```python
from build123d import *

# Parameters (mm, degrees)
F0_R     = 31.75
F1_DEPTH = 12.7
F2_R     = 3
F3_DEPTH = 12.701
F4_R     = 9.95
F5_DEPTH = 12.7
F7_DEPTH = 25.4
F8_R     = 9.525
F9_DEPTH = 19.05


with BuildPart() as f1:
    # F0 (on Top) → F1 (new body)
    with BuildSketch(Plane.XY):
        Circle(F0_R)
    extrude(amount=F1_DEPTH)

    # F2 (on face) → F3 (cut, through all)
    with BuildSketch(Plane.XY.offset(12.7)):
        with Locations((0, 22.5)):
            Circle(F2_R)
        with Locations((-19.485572, 11.25)):
            Circle(F2_R)
        with Locations((-19.485572, -11.25)):
            Circle(F2_R)
        with Locations((0, -22.5)):
            Circle(F2_R)
        with Locations((19.485572, -11.25)):
            Circle(F2_R)
        with Locations((19.485572, 11.25)):
            Circle(F2_R)
    extrude(amount=-F3_DEPTH, mode=Mode.SUBTRACT)

    # F4 (on face) → F5 (cut)
    with BuildSketch(Plane(origin=(0, 0, 0), x_dir=(1, 0, 0), z_dir=(0, 0, -1))):
        Circle(F4_R)
    extrude(amount=-F5_DEPTH, mode=Mode.SUBTRACT)

    # F6 (on face) → F7 (join)
    with BuildSketch(Plane.XY.offset(12.7)):
        with BuildLine():
            ThreePointArc((-4.030746, -18.055556), (0, -16.5), (4.030746, -18.055556))
            ThreePointArc((4.030746, -18.055556), (9.25, -16.02147), (13.621197, -12.518506))
            ThreePointArc((13.621197, -12.518506), (14.289419, -8.25), (17.651943, -5.537049))
            ThreePointArc((17.651943, -5.537049), (18.5, 0), (17.651943, 5.537049))
            ThreePointArc((17.651943, 5.537049), (14.289419, 8.25), (13.621197, 12.518506))
            ThreePointArc((13.621197, 12.518506), (9.25, 16.02147), (4.030746, 18.055556))
            ThreePointArc((4.030746, 18.055556), (0, 16.5), (-4.030746, 18.055556))
            ThreePointArc((-4.030746, 18.055556), (-9.25, 16.02147), (-13.621197, 12.518506))
            ThreePointArc((-13.621197, 12.518506), (-14.289419, 8.25), (-17.651943, 5.537049))
            ThreePointArc((-17.651943, 5.537049), (-18.5, 0), (-17.651943, -5.537049))
            ThreePointArc((-17.651943, -5.537049), (-14.289419, -8.25), (-13.621197, -12.518506))
            ThreePointArc((-13.621197, -12.518506), (-9.25, -16.02147), (-4.030746, -18.055556))
        make_face()
    extrude(amount=F7_DEPTH)

    # F8 (on face) → F9 (cut)
    with BuildSketch(Plane.XY.offset(38.1)):
        Circle(F8_R)
    extrude(amount=-F9_DEPTH, mode=Mode.SUBTRACT)


solid = f1.part
```
Geometry check sheet. Reference: the model listing, model coordinates, mm. A direction names the side the tool comes from. Give positions to 0.01 mm unless a question says otherwise; leave off trailing zeros. Order: outer loops, then holes, each group sorted by start corner. A loop starts at its lowest first (then second) coordinate and runs counter-clockwise, first axis right, second up. Notation, with made-up numbers: (-31.5, 16.5) - (24.5, 16.5) arc R17 cw to (24.5, 21.5) - close; hole circle Ø7 at (13, 28). An arc over 180 degrees is marked (long way). Answer in a Markdown table with one row per item. Add a question column.
Q1. Mould release check, pull along X, two halves, no side actions. Record for faces 4 (the cylindrical face through (14.26, -8.3, 25.22)), 5 (the cylindrical face through (-0.1, -16.5, 25.2)), 6 (the flat face through (-8, -7, 0)), 7 (the cylindrical face through (-22.483, 11.382, 6.439)): pulls with the +X half, pulls with the -X half, needs draft (parallel to the pull), parting line crosses it, or undercut.
Q2. Material ranges on probe 1 along Y at (x, z) = (0, 8.25); probe 2 along Y at (x, z) = (22, 9.5); probe 3 along Z at (x, y) = (13, 23.5), recorded low to high. Write a range as from..to.
Q3. Cross-section at C-C, the plane y = 22.5. Enter the section's corners in (x, z).
Q4. Cross-section at D-D, the plane y = 11.25. Enter the section's corners in (x, z), then the cut area to 3 significant figures.
Q5. Gauge pin test, flat ends, axial feed: pin 1 (6 mm diameter, centred on x = 1, y = -1, fed in from -Z); pin 2 (5 mm diameter, centred on x = -0.5, z = 24, fed in from -Y); pin 3 (7 mm diameter, centred on x = 19.49, y = 11.25, fed in from +Z). Record the tip position at first contact, or that the pin passes through.
Q6. Tool access check on faces 1 (the cylindrical face through (9.18, -16.06, 25.22)), 2 (the cylindrical face through (-7.9, 6.05, 6.26)), 3 (the cylindrical face through (-7.559, -5.796, 28.708)). Record the directions out of +Z, -Z, +X, -X, +Y, -Y that give a thin tool (end or side, any length) a straight path to the whole face; none if there is none.
Q7. Cross-section at B-B, the plane x = 0. Enter the section's corners in (y, z) (3 decimals), then the cut area to 3 significant figures.
Check values:
| question | item | result |
|---|---|---|
| 1 | face 4 | pulls with the +X half |
| 1 | face 5 | undercut |
| 1 | face 6 | needs draft |
| 1 | face 7 | undercut |
| 2 | probe 1 | y = -31.75..-25.5, -19.5..-9.95, 9.95..19.5, 25.5..31.75 |
| 2 | probe 2 | y = -22.89..-12.89, -9.61..9.61, 12.89..22.89 |
| 2 | probe 3 | z = 0..12.7 |
| 3 | outline | (-22.4, 0) - (-3, 0) - (-3, 12.7) - (-22.4, 12.7) - close; (3, 0) - (22.4, 0) - (22.4, 12.7) - (3, 12.7) - close |
| 4 | outline | (-29.69, 0) - (-22.49, 0) - (-22.49, 12.7) - (-29.69, 12.7) - close; (-16.49, 0) - (16.49, 0) - (16.49, 12.7) - (13.49, 12.7) - (13.49, 38.1) - (-13.49, 38.1) - (-13.49, 12.7) - (-16.49, 12.7) - close; (22.49, 0) - (29.69, 0) - (29.69, 12.7) - (22.49, 12.7) - close |
| 4 | area | 1,290 mm^2 |
| 5 | pin 1 | stops at z = 12.7 |
| 5 | pin 2 | stops at y = -17.3 |
| 5 | pin 3 | stops at z = 12.7 |
| 6 | face 1 | +Z, +X, -Y |
| 6 | face 2 | -Z |
| 6 | face 3 | +Z |
| 7 | outline | (-31.75, 0) - (-25.5, 0) - (-25.5, 12.7) - (-31.75, 12.7) - close; (-19.5, 0) - (-9.95, 0) - (-9.95, 12.7) - (9.95, 12.7) - (9.95, 0) - (19.5, 0) - (19.5, 12.7) - (16.5, 12.7) - (16.5, 38.1) - (9.525, 38.1) - (9.525, 19.05) - (-9.525, 19.05) - (-9.525, 38.1) - (-16.5, 38.1) - (-16.5, 12.7) - (-19.5, 12.7) - close; (25.5, 0) - (31.75, 0) - (31.75, 12.7) - (25.5, 12.7) - close |
| 7 | area | 877 mm^2 |
